CAD build for the part. Positions are in the model's coordinates, mm. A direction names the side the tool comes from. Coordinates: 2 decimals unless noted, no trailing zeros. Write each loop counter-clockwise with the first axis right and the second up, starting at its lowest first coordinate (ties: lowest second). Pieces come first, ordered by that corner, then holes.
```python
from build123d import *

# Parameters (mm, degrees)
SKETCH_R        = 9
PAD_DEPTH       = 15
POCKET_DEPTH    = 14
SKETCH002_R     = 7
POCKET001_DEPTH = 2
SKETCH003_R     = 1.5
POCKET002_DEPTH = 9.001
SKETCH004_W     = 1
SKETCH004_H     = 2
CHAMFER_SIZE    = 1
CHAMFER001_SIZE = 0.5


with BuildPart() as part:
    # Sketch → Pad (new body)
    with BuildSketch(Plane.XY):
        Circle(SKETCH_R)
    extrude(amount=PAD_DEPTH)

    # Sketch001 → Pocket (cut)
    with BuildSketch(Plane.XY):
        with BuildLine():
            ThreePointArc((-1.658312, 2.5), (0, -3), (1.658312, 2.5))
            Line((-1.658312, 2.5), (1.658312, 2.5))
        make_face()
    extrude(amount=POCKET_DEPTH, mode=Mode.SUBTRACT)

    # Sketch002 → Pocket001 (cut)
    with BuildSketch(Plane.XY):
        Circle(SKETCH002_R)
    extrude(amount=POCKET001_DEPTH, mode=Mode.SUBTRACT)

    # Sketch003 → Pocket002 (cut, through all)
    with BuildSketch(Plane.XZ):
        with Locations((0, 6)):
            Circle(SKETCH003_R)
    extrude(amount=-POCKET002_DEPTH, mode=Mode.SUBTRACT)

    # Sketch004 → Groove (revolve, cut)
    with BuildSketch(Plane.XZ):
        with Locations((8.5, 14)):
            Rectangle(SKETCH004_W, SKETCH004_H)
        with Locations((8.5, 1)):
            Rectangle(SKETCH004_W, SKETCH004_H)
    revolve(axis=Axis((0, 0, 0), (0, 0, 1)), mode=Mode.SUBTRACT)

    # Chamfer
    chamfer_edges = [part.edges().sort_by_distance(p)[0] for p in [
        (-8, 0, 15),
    ]]
    chamfer(chamfer_edges, length=CHAMFER_SIZE)

    # Chamfer001
    chamfer001_edges = [part.edges().sort_by_distance(p)[0] for p in [
        (-9, 0, 2),
        (9, 0, 7.5),
        (-9, 0, 13),
        (-1.5, 8.87412, 6),
    ]]
    chamfer(chamfer001_edges, length=CHAMFER001_SIZE)


solid = part.part
```
Item 1: Saw through at A-A, the plane z = 10.25. Write the cut outline in (x, y), and give its area (3 significant figures).
Item 2: Which spindle directions (+Z, -Z, +X, -X, +Y, -Y) get a long thin tool onto all of the face, cutting with end or side? Do faces 4 (the cylindrical face through (-0.325, 5.458, 4.536)), 5 (the cylindrical face through (-1.73, -7.81, 13.51)), 6 (the cylindrical face through (6.466, -2.681, 0.986)), 7 (the flat face through (4, -6, 0)). Say none if no direction does.
Item 3: Saw through at B-B, the plane y = 0. Write the cut outline in (x, z), and give its area (4 significant figures).
Item 4: Two-plate mould, pull along Y, no slides. Class faces 1 (the cylindrical face through (-1.951, -8.786, 7.43)), 2 (the cylindrical face through (0, -3, 8)), 3 (the flat face through (0, 0, 15)): +Y half, -Y half, draft (parallel to the pull), parting line (faces both ways), or undercut.
Item 5: Wall check: line 1 along Y through (x, z) = (0, 1.4); line 2 along Z through (x, y) = (0, 5.5); line 3 along Y through (x, z) = (-2.75, 2.75). Give the ranges that are in metal, low to high.
Item 6: Flat gauge pins, fed straight in: pin 1 Ø1.6 at (x, y) = (-1, -1.5) entering from -Z; pin 2 Ø5 at (x, y) = (-0.5, -3.5) entering from -Z; pin 3 Ø1.5 at (x, z) = (5, 6) entering from +Y. Where does each tip first touch, or does it go through?
Working result:
1. outline: circle Ø18 at (0, 0); hole (-1.66, 2.5) arc R3 ccw (long way) to (1.66, 2.5) - close
1. area: 227 mm2
2. face 4: +Y
2. face 5: +Z
2. face 6: -Z
2. face 7: -Z, +X, -X, +Y, -Y
3. outline: (-9, 2.5) - (-8.5, 2) - (-8, 2) - (-8, 0) - (-7, 0) - (-7, 2) - (-3, 2) - (-3, 14) - (3, 14) - (3, 2) - (7, 2) - (7, 0) - (8, 0) - (8, 2) - (8.5, 2) - (9, 2.5) - (9, 12.5) - (8.5, 13) - (8, 13) - (8, 14) - (7, 15) - (-7, 15) - (-8, 14) - (-8, 13) - (-8.5, 13) - (-9, 12.5) - close
3. area: 160.5 mm2
4. face 1: parting line
4. face 2: undercut
4. face 3: draft
5. line 1: y = -8 to -7, 7 to 8
5. line 2: z = 2 to 4.5, 7.5 to 15
5. line 3: y = -8.57 to -1.2, 1.2 to 8.57
6. pin 1: stops at z = 14
6. pin 2: stops at z = 2
6. pin 3: stops at y = 7.93
